```python
from build123d import *

# Parameters (mm, degrees)
F0_W          = 6.1
F0_H          = 4.39
F0_R          = 0.25
F1_DEPTH      = 4.65
F2_DEPTH      = 4.65
F2_DEPTH_BACK = 12.7


with BuildPart() as f1:
    # F0 (on Top) → F1 (new body)
    with BuildSketch(Plane.XY):
        Rectangle(F0_W, F0_H)
        with Locations((-1.27, -1.055)):
            Circle(F0_R, mode=Mode.SUBTRACT)
        with Locations((1.27, -1.055)):
            Circle(F0_R, mode=Mode.SUBTRACT)
        with Locations((-1.27, 1.055)):
            Circle(F0_R, mode=Mode.SUBTRACT)
        with Locations((1.27, 1.055)):
            Circle(F0_R, mode=Mode.SUBTRACT)
    extrude(amount=F1_DEPTH)

    # F0 (on Top) → F2 (join, two sides)
    with BuildSketch(Plane.XY) as f2_sk:
        with Locations((1.27, 1.055)):
            Circle(F0_R)
        with Locations((-1.27, 1.055)):
            Circle(F0_R)
        with Locations((1.27, -1.055)):
            Circle(F0_R)
        with Locations((-1.27, -1.055)):
            Circle(F0_R)
    extrude(amount=F2_DEPTH)
    extrude(f2_sk.sketch, amount=-F2_DEPTH_BACK)


solid = f1.part
```
Verification items for the finished model (mm, model axes). A direction names the side the tool comes from. Coordinates: 2 decimals unless noted, no trailing zeros. Order: outer loops, then holes, each group sorted by start corner. A loop starts at its lowest first (then second) coordinate and runs counter-clockwise, first axis right, second up. Notation, with made-up numbers: (-29, -36.5) -> (-22, -36.5) arc R12 cw to (-22, -32.5) -> close; hole circle Ø10 at (1.5, 89.25). An arc over 180 degrees is marked (long way). Put each result on its own line as item: value. Start each with the question number.
1) Cross-section at C-C (z = -2.25). Enter the section's corners in (x, y) (3 decimals).
2) Cross-section at D-D (x = 2). Enter the section's corners in (y, z) (3 decimals).
3) Cross-section at B-B (y = 1.7). Enter the section's corners in (x, z), plus the area to 3 significant figures.
4) Tool access check on faces 1 (the flat face through (0, -2.195, 2)), 2 (the flat face through (0, 0, 0)). Record the directions out of +Z, -Z, +X, -X, +Y, -Y that give a thin tool (end or side, any length) a straight path to the whole face; none if there is none.
5) Cross-section at A-A (x = 1.27). Enter the section's corners in (y, z) (3 decimals).
6) Material ranges on L1, parallel to Y at x = 1.25, z = -11.25; L2, parallel to X at y = 0.95, z = -10.25; L3, parallel to Z at x = 1, y = 1.25, recorded low to high.
Geometry check:
1. outline: circle Ø0.5 at (-1.27, -1.055); circle Ø0.5 at (-1.27, 1.055); circle Ø0.5 at (1.27, -1.055); circle Ø0.5 at (1.27, 1.055)
2. outline: (-2.195, 0) -> (2.195, 0) -> (2.195, 4.65) -> (-2.195, 4.65) -> close
3. outline: (-3.05, 0) -> (3.05, 0) -> (3.05, 4.65) -> (-3.05, 4.65) -> close
3. area: 28.4 mm^2
4. face 1: +Z, -Z, +X, -X, -Y
4. face 2: -Z
5. outline: (-2.195, 0) -> (-1.305, 0) -> (-1.305, -12.7) -> (-0.805, -12.7) -> (-0.805, 0) -> (0.805, 0) -> (0.805, -12.7) -> (1.305, -12.7) -> (1.305, 0) -> (2.195, 0) -> (2.195, 4.65) -> (-2.195, 4.65) -> close
6. L1: y = -1.3 to -0.81, 0.81 to 1.3
6. L2: x = -1.5 to -1.04, 1.04 to 1.5
6. L3: z = 0 to 4.65
